Verification items for the finished model (mm, model axes). Face numbers are marked on the shaded views. A direction names the side the tool comes from. Give positions to 0.01 mm unless a question says otherwise; leave off trailing zeros. Write each loop counter-clockwise with the first axis right and the second up, starting at its lowest first coordinate (ties: lowest second). Pieces come first, ordered by that corner, then holes. Notation, with made-up numbers: M -39,6.25 L 1,6.25 A18 cw 1,35.25 Z; hole C 75,63 d10. An arc over 180 degrees is marked long. Answer as a JSON object with one key per item and string values.
```python
from build123d import *

# Parameters (mm, degrees)
SKETCH1_W                 = 55.88
SKETCH1_H                 = 40.64
BOSS_EXTRUDE1_DEPTH       = 25.4
SKETCH3_R                 = 3.81
CUT_EXTRUDE1_DEPTH        = 41.64
M5X0_8_TAPPED_HOLE1_D     = 4.2
M5X0_8_TAPPED_HOLE1_DEPTH = 25.4
M5X0_8_TAPPED_HOLE1_TIP   = 1.2618073
CUT_EXTRUDE3_DEPTH        = 15.732509398
CUT_EXTRUDE3_DEPTH_BACK   = 25.26481483


with BuildPart() as part:
    # Sketch1 → Boss-Extrude1 (new body)
    with BuildSketch(Plane(origin=(0, 0, 0), x_dir=(1, 0, 0), z_dir=(0, 1, 0))):
        with Locations((27.94, 20.32)):
            Rectangle(SKETCH1_W, SKETCH1_H)
    extrude(amount=BOSS_EXTRUDE1_DEPTH)

    # Sketch3 → Cut-Extrude1 (cut, through all)
    with BuildSketch(Plane.XY):
        with Locations((9.525, 12.7)):
            Circle(SKETCH3_R)
    extrude(amount=-CUT_EXTRUDE1_DEPTH, mode=Mode.SUBTRACT)

    # M5x0.8 Tapped Hole1
    with Locations(Plane.XY):
        with Locations((50.8, 5.08), (33.02, 5.08), (33.02, 20.32), (50.8, 20.32)):
            Hole(M5X0_8_TAPPED_HOLE1_D / 2, depth=M5X0_8_TAPPED_HOLE1_DEPTH)
            with Locations((0, 0, -(M5X0_8_TAPPED_HOLE1_DEPTH + M5X0_8_TAPPED_HOLE1_TIP / 2))):  # 118° drill point
                Cone(0, M5X0_8_TAPPED_HOLE1_D / 2, M5X0_8_TAPPED_HOLE1_TIP, mode=Mode.SUBTRACT)

    # Sketch8 → Cut-Extrude3 (cut, two sides)
    with BuildSketch(Plane(origin=(-2.536945986, 9.468011314, 0), x_dir=(0.965925826, 0.258819045, 0), z_dir=(-0.258819045, 0.965925826, 0))) as cut_extrude3_sk:
        with BuildLine():
            ThreePointArc((11.137445368, 20.19), (4.787445368, 26.54), (11.137445368, 32.89))
            Line((11.137445368, 32.89), (0, 32.89))
            Line((0, 32.89), (0, 20.19))
            Line((0, 20.19), (11.137445368, 20.19))
        make_face()
        with BuildLine():
            ThreePointArc((17.487445368, 26.54), (15.627573429, 31.030128061), (11.137445368, 32.89))
            Line((11.137445368, 32.89), (11.137445368, 20.19))
            ThreePointArc((11.137445368, 20.19), (15.627573429, 22.049871939), (17.487445368, 26.54))
        make_face()
        with BuildLine():
            Line((11.137445368, 20.19), (11.137445368, 32.89))
            ThreePointArc((11.137445368, 32.89), (4.787445368, 26.54), (11.137445368, 20.19))
        make_face()
    extrude(amount=CUT_EXTRUDE3_DEPTH, mode=Mode.SUBTRACT)
    extrude(cut_extrude3_sk.sketch, amount=-CUT_EXTRUDE3_DEPTH_BACK, mode=Mode.SUBTRACT)


solid = part.part
```
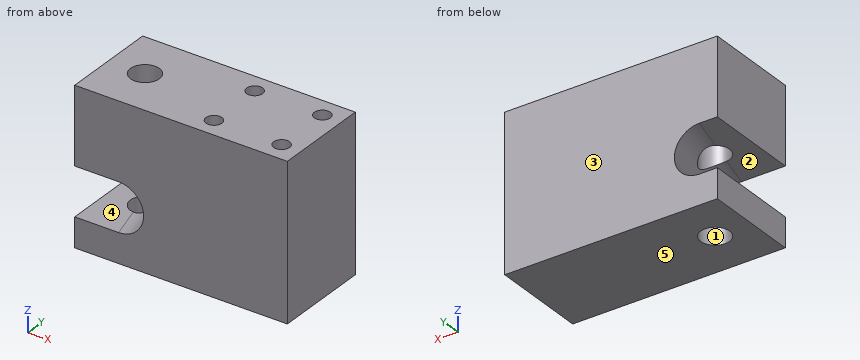
1) Access from +Z, -Z, +X, -X, +Y, -Y to the whole of each face (thin tool, end or side, straight path). Record for the marked faces 4 and 5.
Completed:
{"face 4": "-X, -Y", "face 5": "-Z, +X, -X, +Y, -Y"}
2) Release check for a two-part mould opening along Y. For the marked faces 1, 2 and 3 record: pulls with the +Y half, pulls with the -Y half, needs draft (parallel to the pull), parting line crosses it, or undercut.
Completed:
{"face 1": "undercut", "face 2": "needs draft", "face 3": "pulls with the +Y half"}
3) Thickness scan on L1, parallel to Y at x = 50.8, z = -16; L2, parallel to X at y = 5.08, z = -19.5; L3, parallel to X at y = 5.5, z = -4. Record the ranges inside material, lowest first.
Completed:
{"L1": "y = 0 to 2.98, 7.18 to 18.22, 22.42 to 25.4", "L2": "x = 0 to 30.92, 35.12 to 48.7, 52.9 to 55.88", "L3": "x = 0 to 30.96, 35.08 to 48.74, 52.86 to 55.88"}
4) Section check B-B on x = 8. Count the separate pieces of the cut face and the enclosed holes in it, and give its area (3 significant figures).
Completed:
{"separate pieces": "4", "enclosed holes": "0", "area": "521 mm2"}
5) Section check A-A on z = -17.5. Record the boundary of the cut face in (x, y) (3 decimals).
Completed:
{"outline": "M 0,0 L 55.88,0 L 55.88,25.4 L 0,25.4 Z; hole C 9.525,12.7 d7.62; hole C 33.02,5.08 d4.2; hole C 33.02,20.32 d4.2; hole C 50.8,5.08 d4.2; hole C 50.8,20.32 d4.2"}
